Build history of the part. All positions in model axes, mm. Face numbers are marked on the shaded views. Round coordinates to 2 decimals unless told otherwise and drop trailing zeros. Loops run counter-clockwise (first coordinate to the right, second up) from the corner with the lowest first, then second, coordinate; pieces in that order, holes last. Notation, with made-up numbers: (-38, 76.25) - (21, 76.25) arc R17 ccw to (21, 85.25) - close; hole circle Ø2 at (41, 54). An arc over 180 degrees is marked (long way). Use a Markdown table: item, result.
from build123d import *

# Parameters (mm, degrees)
SKETCH1_W              = 18.25
SKETCH1_H              = 25
BOSS_EXTRUDE1_DEPTH    = 8
M10X1_0_TAPPED_HOLE1_D = 9
SKETCH7_R              = 3.375
SKETCH7_R_2            = 0.9906
CUT_EXTRUDE2_DEPTH     = 19.25


with BuildPart() as part:
    # Sketch1 → Boss-Extrude1 (new body)
    with BuildSketch(Plane(origin=(0, 0, 0), x_dir=(1, 0, 0), z_dir=(0, 1, 0))):
        with Locations((0, -5.5)):
            Rectangle(SKETCH1_W, SKETCH1_H)
    extrude(amount=BOSS_EXTRUDE1_DEPTH)

    # M10x1.0 Tapped Hole1 (through all)
    with Locations(Plane(origin=(0, 8, 0), x_dir=(-1, 0, 0), z_dir=(0, 1, 0))):
        with Locations((0, 0)):
            Hole(M10X1_0_TAPPED_HOLE1_D / 2)

    # Sketch7 → Cut-Extrude2 (cut, through all)
    with BuildSketch(Plane(origin=(9.125, 0, 0), x_dir=(0, 0, -1), z_dir=(1, 0, 0))):
        with Locations((-13.336186812, 4)):
            Circle(SKETCH7_R)
        with Locations((-7.3575, 4)):
            Circle(SKETCH7_R_2)
    extrude(amount=-CUT_EXTRUDE2_DEPTH, mode=Mode.SUBTRACT)


solid = part.part
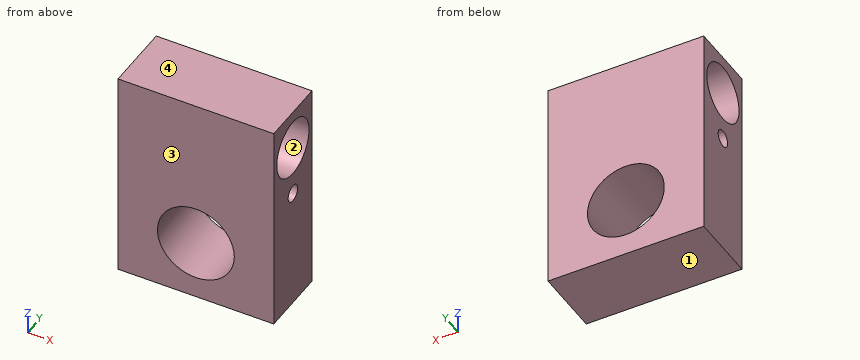
Q1. Cut at B-B, the plane x = 0. Count the separate pieces of the cut face and the enclosed holes in it, plus the area to 3 significant figures.
Results found:
| item | result |
|---|---|
| separate pieces | 2 |
| enclosed holes | 2 |
| area | 89.1 mm2 |
Q2. Pull direction Z, two halves, no side cores. Call the marked faces 1, 2, 3 and 4: pulls with the +Z half, pulls with the -Z half, needs draft (parallel to the pull), parting line crosses it, or undercut.
Results found:
| item | result |
|---|---|
| face 1 | pulls with the -Z half |
| face 2 | undercut |
| face 3 | needs draft |
| face 4 | pulls with the +Z half |
Q3. Cut at C-C, the plane z = 0. List the corners of the cut face in (x, y) (3 decimals).
Results found:
| item | result |
|---|---|
| outline | (-9.125, 0) - (-4.5, 0) - (-4.5, 8) - (-9.125, 8) - close; (4.5, 0) - (9.125, 0) - (9.125, 8) - (4.5, 8) - close |
Q4. Cut at A-A, the plane y = 4. List the corners of the cut face in (x, z) (3 decimals), plus the area to 3 significant figures.
Results found:
| item | result |
|---|---|
| outline | (-9.125, -7) - (9.125, -7) - (9.125, 6.367) - (-9.125, 6.367) - close; (-9.125, 8.348) - (9.125, 8.348) - (9.125, 9.961) - (-9.125, 9.961) - close; (-9.125, 16.711) - (9.125, 16.711) - (9.125, 18) - (-9.125, 18) - close; hole circle Ø9 at (0, 0) |
| area | 233 mm2 |
Q5. Probe line 1 (Y direction, x = 6.5, z = 13.5); line 2 (Z direction, x = 3.25, y = 7); line 3 (Z direction, x = 0, y = 6.25). List the from-to ranges inside material, lowest first.
Results found:
| item | result |
|---|---|
| line 1 | y = 0 to 0.63, 7.37 to 8 |
| line 2 | z = -7 to -3.11, 3.11 to 11.79, 14.88 to 18 |
| line 3 | z = -7 to -4.5, 4.5 to 10.82, 15.85 to 18 |
Q6. Drop a flat-ended pin along its axis: pin 1 (8 mm diameter, centred on x = 0, z = 0, fed in from -Y). Give the stop position or say it passes through.
Results found:
| item | result |
|---|---|
| pin 1 | passes through |
